```python
from build123d import *

# Parameters (mm, degrees)
SKETCH_1_R      = 1.5
EXTRUDE_1_DEPTH = 3
FILLET_1_R      = 2.5
FILLET_2_R      = 1


with BuildPart() as part:
    # Эскиз1 → Бобышка-Вытянуть1 (new body)
    with BuildSketch(Plane.XY):
        Polygon((-60, 17.5), (-60, 0), (-66.8, 0), (-66.8, 17.5), (-70.8, 17.5), (-70.8, -17.5), (70.8, -17.5), (70.8, 17.5), (66.8, 17.5), (66.8, 0), (60, 0), (60, 17.5), align=None)
        with BuildLine():
            Line((48, -12.5), (-48, -12.5))
            ThreePointArc((-48, -12.5), (-49.318019485, -9.318019485), (-52.5, -8))
            Line((-52.5, -8), (-52.5, 8))
            ThreePointArc((-52.5, 8), (-49.318019485, 9.318019485), (-48, 12.5))
            Line((-48, 12.5), (48, 12.5))
            ThreePointArc((48, 12.5), (49.318019485, 9.318019485), (52.5, 8))
            Line((52.5, 8), (52.5, -8))
            ThreePointArc((52.5, -8), (49.318019485, -9.318019485), (48, -12.5))
        make_face(mode=Mode.SUBTRACT)
        with Locations((-52.5, 12.5)):
            Circle(SKETCH_1_R, mode=Mode.SUBTRACT)
        with Locations((-52.5, -12.5)):
            Circle(SKETCH_1_R, mode=Mode.SUBTRACT)
        with Locations((52.5, -12.5)):
            Circle(SKETCH_1_R, mode=Mode.SUBTRACT)
        with Locations((52.5, 12.5)):
            Circle(SKETCH_1_R, mode=Mode.SUBTRACT)
    extrude(amount=EXTRUDE_1_DEPTH)

    # Скругление1
    fillet_1_edges = [part.edges().sort_by_distance(p)[0] for p in [
        (-70.8, -17.5, 1.5),
        (70.8, -17.5, 1.5),
    ]]
    fillet(fillet_1_edges, radius=FILLET_1_R)

    # Скругление2
    fillet_2_edges = [part.edges().sort_by_distance(p)[0] for p in [
        (-70.8, 17.5, 1.5),
        (-66.8, 17.5, 1.5),
        (-60, 17.5, 1.5),
        (60, 17.5, 1.5),
        (66.8, 17.5, 1.5),
        (70.8, 17.5, 1.5),
    ]]
    fillet(fillet_2_edges, radius=FILLET_2_R)


solid = part.part
```
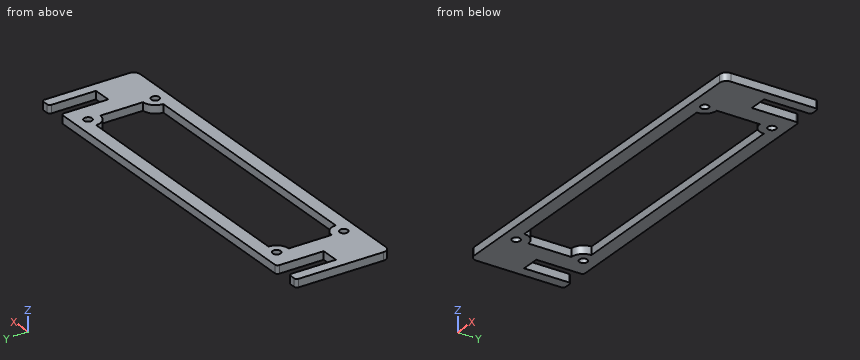
Geometry: final body of the model. Coordinates: model frame, mm. Round coordinates to 2 decimals unless told otherwise and drop trailing zeros. Order: outer loops, then holes, each group sorted by start corner. A loop starts at its lowest first (then second) coordinate and runs counter-clockwise, first axis right, second up. Notation, with made-up numbers: (28.5, 36) -> (62.5, 36) arc R24 ccw to (62.5, 72) -> close; hole circle Ø9 at (-23, 3.25). An arc over 180 degrees is marked (long way). Use one line per item in the form item = value. Start each with the question number.
1. Pin query (flat end, axial travel): pin 1 Ø0.9 at (x, z) = (64.5, 1) entering from +Y; pin 2 Ø2.5 at (x, y) = (52.5, -12.5) entering from +Z. Return the tip coordinate at first contact, or that it passes through.
2. Line query: probe 1 along X at (y, z) = (15, 0.9); probe 2 along X at (y, z) = (3.5, 0.35); probe 3 along X at (y, z) = (-12, 1.85). Output: solid intervals per line, ascending.
3. Cut plane B-B (z = 2.2). Count the separate pieces of the cut face and the enclosed holes in it, then the cut area to 3 significant figures.
4. Cut plane A-A (x = 29.5). Return the cut outline in (y, z).
Solution:
q1.pin_1 = 0
q1.pin_2 = through
q2.probe_1 = -70.8 to -66.8, -60 to 60, 66.8 to 70.8
q2.probe_2 = -70.8 to -66.8, -60 to -52.5, 52.5 to 60, 66.8 to 70.8
q2.probe_3 = -70.8 to -53.91, -51.09 to -48.03, 48.03 to 51.09, 53.91 to 70.8
q3.separate_pieces = 1
q3.enclosed_holes = 5
q3.area = 2,120 mm^2
q4.outline = (-17.5, 0) -> (-12.5, 0) -> (-12.5, 3) -> (-17.5, 3) -> close; (12.5, 0) -> (17.5, 0) -> (17.5, 3) -> (12.5, 3) -> close
